```python
from build123d import *

# Parameters (mm, degrees)
ESQUISSE1_W        = 230
ESQUISSE1_H        = 30
BOSS_EXTRU_1_DEPTH = 2
ESQUISSE2_R        = 7.5
ESQUISSE2_R_2      = 5
BOSS_EXTRU_2_DEPTH = 3


with BuildPart() as part:
    # Esquisse1 → Boss.-Extru.1 (new body)
    with BuildSketch(Plane.XY):
        with Locations((115, 15)):
            Rectangle(ESQUISSE1_W, ESQUISSE1_H)
    extrude(amount=BOSS_EXTRU_1_DEPTH)

    # Esquisse2 → Boss.-Extru.2 (add)
    # profile 1 of 5: a face of its own
    with BuildSketch(Plane.XY.offset(2)):
        with Locations(Location((15, 15, 0), (0, 0, 180))):
            Circle(ESQUISSE2_R)
        with Locations((15, 15)):
            Circle(ESQUISSE2_R_2, mode=Mode.SUBTRACT)
    # profile 2 of 5: a face of its own
    with BuildSketch(Plane.XY.offset(2)):
        with Locations(Location((65, 15, 0), (0, 0, 180))):
            Circle(ESQUISSE2_R)
        with Locations((65, 15)):
            Circle(ESQUISSE2_R_2, mode=Mode.SUBTRACT)
    # profile 3 of 5: a face of its own
    with BuildSketch(Plane.XY.offset(2)):
        with Locations(Location((115, 15, 0), (0, 0, 180))):
            Circle(ESQUISSE2_R)
        with Locations((115, 15)):
            Circle(ESQUISSE2_R_2, mode=Mode.SUBTRACT)
    # profile 4 of 5: a face of its own
    with BuildSketch(Plane.XY.offset(2)):
        with Locations(Location((165, 15, 0), (0, 0, 180))):
            Circle(ESQUISSE2_R)
        with Locations((165, 15)):
            Circle(ESQUISSE2_R_2, mode=Mode.SUBTRACT)
    # profile 5 of 5: a face of its own
    with BuildSketch(Plane.XY.offset(2)):
        with Locations(Location((215, 15, 0), (0, 0, 180))):
            Circle(ESQUISSE2_R)
        with Locations((215, 15)):
            Circle(ESQUISSE2_R_2, mode=Mode.SUBTRACT)
    extrude(amount=BOSS_EXTRU_2_DEPTH)


solid = part.part
```
CAD build for the part. Positions are in the model's coordinates, mm. A direction names the side the tool comes from. Round coordinates to 2 decimals unless told otherwise and drop trailing zeros. Write each loop counter-clockwise with the first axis right and the second up, starting at its lowest first coordinate (ties: lowest second). Pieces come first, ordered by that corner, then holes. Notation, with made-up numbers: M 49.5,-28 L 55.5,-28 A25 ccw 55.5,-11 Z; hole C 82.5,86 d2. An arc over 180 degrees is marked long. One line per question, with ' | ' between items.
1. Cut at A-A on x = 65. Write the cut outline in (y, z).
Working result:
outline: M 0,0 L 30,0 L 30,2 L 22.5,2 L 22.5,5 L 20,5 L 20,2 L 10,2 L 10,5 L 7.5,5 L 7.5,2 L 0,2 Z
2. Mould opens along X. For faces 1 (the flat face through (65, 15, 2)), 2 (the flat face through (113, 20, 5)) say: pulls with the +X half, pulls with the -X half, needs draft (parallel to the pull), parting line crosses it, or undercut.
Working result:
face 1: undercut | face 2: needs draft
3. Cut at C-C on x = 144.5. Write the cut outline in (y, z).
Working result:
outline: M 0,0 L 30,0 L 30,2 L 0,2 Z
4. Pin check, flat tips, straight feed: pin 1 Ø8 at (x, y) = (75.5, 22.5) entering from +Z; pin 2 Ø11 at (x, y) = (215, 16) entering from +Z. Stop position of each tip, or through.
Working result:
pin 1: z = 2 | pin 2: z = 5
5. Cut at B-B on y = 24.5. Write the cut outline in (x, z).
Working result:
outline: M 0,0 L 230,0 L 230,2 L 0,2 Z
6. Probe L1, parallel to Y at x = 215, z = 2.7; L2, parallel to Z at x = 101, y = 2; L3, parallel to Y at x = 117, z = 4. List the from-to ranges inside material, lowest first. Write a range as from..to.
Working result:
L1: 7.5..10, 20..22.5 | L2: 0..2 | L3: 7.77..10.42, 19.58..22.23
7. Which spindle directions (+Z, -Z, +X, -X, +Y, -Y) get a long thin tool onto all of the face, cutting with end or side? Do faces 3 (the cylindrical face through (70.5, 9.9, 3.5)), 4 (the flat face through (113, 15, 0)). Say none if no direction does.
Working result:
face 3: +Z | face 4: -Z, +X, -X, +Y, -Y
